Autodesk Inventor part; units mm, degrees
ref_plane "YZ Plane" through (0, 0, 0) normal (1, 0, 0) x (0, 1, 0)
ref_plane "XZ Plane" through (0, 0, 0) normal (0, 1, 0) x (-1, 0, 0)
ref_plane "XY Plane" through (0, 0, 0) normal (0, 0, 1) x (1, 0, 0)
sketch "Szkic1" plane through (0, 0, 0) normal (0, 1, 0) x (-1, 0, 0)
  point P0 (0, 0)
sketch "Szkic2" plane through (0, 0, 0) normal (0, 1, 0) x (-1, 0, 0)
  line L0 (0, 0) -> (-15, 0)
  line L1 (-15, 0) -> (-15, 100)
  line L2 (-15, 100) -> (0, 100)
  line L3 (0, 100) -> (0, 0)
  line L4 (-7.5, 100) -> (-7.5, 90) construction
  line L5 (-7.5, 0) -> (-7.5, 10) construction
  circle A0 centre (-7.5, 90) radius 1.5
  circle A1 centre (-7.5, 10) radius 1.5
  line L6 (-15, 100) -> (-220, 100)
  line L7 (-220, 100) -> (-220, 92)
  line L8 (-220, 92) -> (-15, 92)
  line L9 (-15, 92) -> (-15, 100)
  line L10 (-15, 0) -> (-220, 0)
  line L11 (-220, 0) -> (-220, 8)
  line L12 (-220, 8) -> (-15, 8)
  line L13 (-15, 8) -> (-15, 0)
  line L14 (-15, 92) -> (-19, 92) construction
  line L15 (-15, 92) -> (-15, 88) construction
  line L16 (-220, 8) -> (-216, 8) construction
  line L17 (-220, 8) -> (-210, 8)
  line L18 (-210, 8) -> (-210, 92)
  line L19 (-210, 92) -> (-220, 92)
  line L20 (-220, 92) -> (-220, 8)
  line L21 (-210, 8) -> (-206, 8) construction
  line L22 (-210, 8) -> (-210, 12) construction
  line L23 (-15, 88) -> (-206, 8)
  line L24 (-19, 92) -> (-210, 12)
  line L25 (-15, 8) -> (-15, 12) construction
  line L26 (-15, 8) -> (-19, 8) construction
  line L27 (-210, 92) -> (-206, 92) construction
  line L28 (-210, 92) -> (-210, 88) construction
  line L29 (-210, 88) -> (-19, 8)
  line L30 (-15, 12) -> (-206, 92)
  line L31 (-220, 96) -> (-205, 96) construction
  line L32 (-220, 4) -> (-205, 4) construction
  circle A2 centre (-205, 96) radius 1.5
  circle A3 centre (-205, 4) radius 1.5
  line L33 (-205, 96) -> (-180, 96) construction
  line L34 (-205, 4) -> (-180, 4) construction
  circle A4 centre (-180, 96) radius 1.5
  circle A5 centre (-180, 4) radius 1.5
  line L35 (-220, 100) -> (-95, 100) construction
  line L36 (-95.6423, 92) -> (-105.6423, 92)
  line L37 (-105.6423, 92) -> (-105.6423, 8)
  line L38 (-105.6423, 8) -> (-95.6423, 8)
  line L39 (-95.6423, 8) -> (-95.6423, 92)
  line L40 (-220, 0) -> (-157.5, 0) construction
  line L41 (-157.5, 8) -> (-147.5, 8)
  line L42 (-147.5, 8) -> (-147.5, 92)
  line L43 (-147.5, 92) -> (-157.5, 92)
  line L44 (-157.5, 92) -> (-157.5, 8)
  point P0 (-105.725, 50)
  point P1 (-105.6423, 50.0346)
  point P2 (-105.6423, 49.9654)
  point P3 (-112.5, 52.8377)
  point P4 (-147.5, 67.4974)
  point P5 (-105.6423, 55.71)
  point P6 (-119.275, 50)
  point P7 (-147.5, 38.178)
  point P8 (-147.5, 61.822)
  point P9 (-112.5, 47.1623)
  point P10 (-105.6423, 44.29)
  point P11 (-147.5, 32.5026)
  point P12 (-157.5, 66.0105)
  point P13 (-157.5, 33.9895)
  point P14 (-157.5, 28.3141)
  point P15 (-157.5, 71.6859)
  point P16 (-95.6423, 59.8985)
  point P17 (-95.6423, 45.7769)
  point P18 (-95.6423, 54.2231)
  point P19 (-95.6423, 40.1015)
  dimension "d0" = 15
  dimension "d1" = 100
  dimension "d2" = 10
  dimension "d3" = 10
  dimension "d4" = 3
  dimension "d5" = 3
  dimension "d6" = 205
  dimension "d7" = 8
  dimension "d8" = 205
  dimension "d9" = 8
  dimension "d10" = 4
  dimension "d11" = 4
  dimension "d12" = 4
  dimension "d13" = 10
  dimension "d14" = 4
  dimension "d15" = 4
  dimension "d16" = 4
  dimension "d17" = 4
  dimension "d18" = 207.0773
  dimension "d19" = 15
  dimension "d20" = 15
  dimension "d21" = 3
  dimension "d22" = 3
  dimension "d23" = 25
  dimension "d24" = 3
  dimension "d25" = 3
  dimension "d26" = 125
  dimension "d27" = 10
  dimension "d28" = 10
extrude "Wyciągnięcie proste1" add sketch "Szkic2" along normal blind 3 contours L0 L1 L2 L3 | L10 L11 L12 L1 | L12 L29 L39 L30 L1 | L1 L8 L7 L6 | L20 L8 L18 L12 | L1 L23 L39 L24 L8 | L39 L29 L37 L30 | L30 L37 L23 L39 | L12 L37 L29 L39 | L18 L24 L44 L23 L12 | L23 L37 L24 L39 | L37 L29 L23 L30 | L30 L23 L37 | L8 L30 L44 L29 L18 | L39 L24 L37 L8 | L23 L30 L24 L37 | L23 L29 L24 L30 | L12 L44 L23 L42 | L23 L42 L24 L29 | L44 L24 L42 L23 | L44 L29 L42 L24 | L24 L29 L42 L30 | L44 L30 L42 L29 | L8 L42 L30 L44
properties part number "lf-esp"
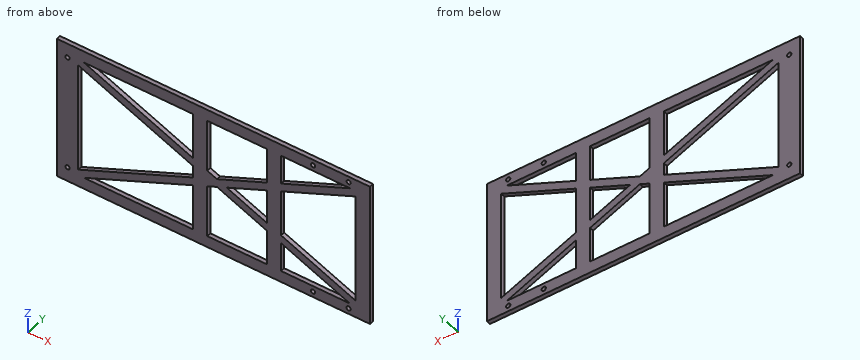
CAD build for the part. Positions are in the model's coordinates, mm. Round coordinates to 2 decimals unless told otherwise and drop trailing zeros. Write each loop counter-clockwise with the first axis right and the second up, starting at its lowest first coordinate (ties: lowest second). Pieces come first, ordered by that corner, then holes. Notation, with made-up numbers: (13, 88.25) - (46, 88.25) arc R22 cw to (46, 116.25) - close; hole circle Ø8 at (7.5, -29.75). An arc over 180 degrees is marked (long way). Write item = value, one per line. Start each with the question number.
Q1. Band-saw the part on C-C (y = 0.75). Count the separate pieces of the cut face and the enclosed holes in it, then the cut area to 3 significant figures.
Q2. Probe L1, parallel to X at y = 1.4, z = 96; L2, parallel to Z at x = 7.5, y = 2.15; L3, parallel to Z at x = 94, y = 0.85. List the from-to ranges inside material, lowest first. Write a range as from..to.
Q3. Band-saw the part on A-A (z = 82.5). Give the cut face in (x, y), then the cut area to 3 significant figures.
Q4. Drop a flat-ended pin along its axis: pin 1 (5 mm diameter, centred on x = 180, z = 4, fed in from -Y). Give the stop position or say it passes through.
Q5. Band-saw the part on B-B (x = 136.5). Give the cut face in (y, z), then the cut area to 3 significant figures.
Answers below:
q1.separate_pieces = 1
q1.enclosed_holes = 15
q1.area = 9,190 mm2
q2.L1 = 0..178.5, 181.5..203.5, 206.5..220
q2.L2 = 0..8.5, 11.5..88.5, 91.5..100
q2.L3 = 0..8, 39.41..45.09, 54.91..60.59, 92..100
q3.outline = (0, 0) - (15, 0) - (15, 3) - (0, 3) - close; (28.13, 0) - (41.68, 0) - (41.68, 3) - (28.13, 3) - close; (95.64, 0) - (105.64, 0) - (105.64, 3) - (95.64, 3) - close; (147.5, 0) - (157.5, 0) - (157.5, 3) - (147.5, 3) - close; (183.32, 0) - (196.87, 0) - (196.87, 3) - (183.32, 3) - close; (210, 0) - (220, 0) - (220, 3) - (210, 3) - close
q3.area = 216 mm2
q4.pin_1 = 0
q5.outline = (0, 0) - (3, 0) - (3, 8) - (0, 8) - close; (0, 37.11) - (3, 37.11) - (3, 42.79) - (0, 42.79) - close; (0, 57.21) - (3, 57.21) - (3, 62.89) - (0, 62.89) - close; (0, 92) - (3, 92) - (3, 100) - (0, 100) - close
q5.area = 82.1 mm2
